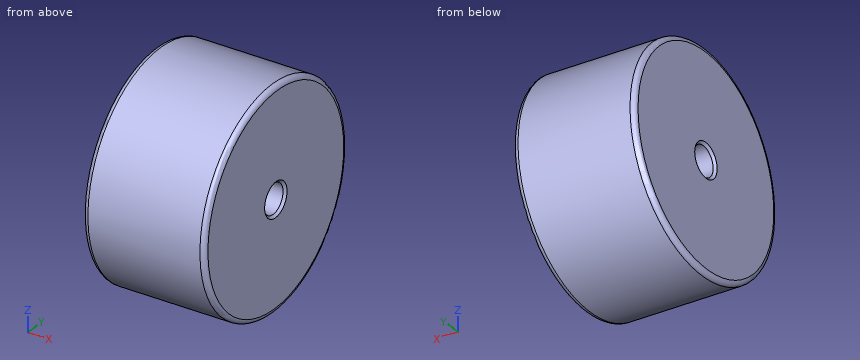
Autodesk Inventor part; units mm, degrees
ref_plane "YZ Plane" through (0, 0, 0) normal (1, 0, 0) x (0, 1, 0)
ref_plane "XZ Plane" through (0, 0, 0) normal (0, 1, 0) x (-1, 0, 0)
ref_plane "XY Plane" through (0, 0, 0) normal (0, 0, 1) x (1, 0, 0)
sketch "Sketch1" plane through (0, 0, 0) normal (1, 0, 0) x (0, 1, 0)
  circle A0 centre (0, 0) radius 45
  circle A1 centre (0, 0) radius 6.1
  dimension "d0" = 90
  dimension "d1" = 12.2
extrude "Extrusion1" add sketch "Sketch1" along normal blind 50
chamfer "Chamfer1" distance 1 angle 45 2 edges at (50, -6.1, 0) (0, -6.1, 0)
fillet "Fillet1" radius 2 2 edges at (0, -45, 0) (50, -45, 0)
properties part number "ciezarek" material "Iron, Cast"
Design review of the part built by this model. Coordinates are the model's own, in mm. Give positions to 0.01 mm unless a question says otherwise; leave off trailing zeros. Order: outer loops, then holes, each group sorted by start corner. A loop starts at its lowest first (then second) coordinate and runs counter-clockwise, first axis right, second up. Notation, with made-up numbers: (7, 41) - (49, 41) arc R34 cw to (49, 75) - close; hole circle Ø9 at (39.25, 36). An arc over 180 degrees is marked (long way). Use a Markdown table: item, result. Add a question column.
(1) Add section A-A on z = 0. Give the boundary of the cut face in (x, y).
(2) Add section C-C on x = 12. Give the boundary of the cut face in (y, z).
(3) Clearance check with flat-ended pins moving along their axes: P1, Ø1.5, axis at x = 28.5, y = -33.5, coming from the -Z side; P2, Ø2, axis at x = 22, z = -30, coming from the -Y side; P3, Ø1.5, axis at y = 28, z = -35, coming from the -X side. State where each tip first meets the part, or that it passes through.
(4) Wall thickness on probe 1 along Z at (x, y) = (26, 0); probe 2 along Y at (x, z) = (32, 4); probe 3 along X at (y, z) = (-31.5, 29.5): over which ranges is each line inside the solid? List them lowest first. Write a range as [from, to].
Report:
| question | item | result |
|---|---|---|
| 1 | outline | (0, -43) arc R2 ccw to (2, -45) - (48, -45) arc R2 ccw to (50, -43) - (50, -7.1) - (49, -6.1) - (1, -6.1) - (0, -7.1) - close; (0, 7.1) - (1, 6.1) - (49, 6.1) - (50, 7.1) - (50, 43) arc R2 ccw to (48, 45) - (2, 45) arc R2 ccw to (0, 43) - close |
| 2 | outline | circle Ø90 at (0, 0); hole circle Ø12.2 at (0, 0) |
| 3 | P1 | stops at z = -30.86 |
| 3 | P2 | stops at y = -34.41 |
| 3 | P3 | stops at x = 0.31 |
| 4 | probe 1 | z = [-45, -6.1], [6.1, 45] |
| 4 | probe 2 | y = [-44.82, -4.61], [4.61, 44.82] |
| 4 | probe 3 | x = [0.01, 49.99] |
